Read the model definition and answer for the solid it produces. Units are mm, in the model's axes. A direction names the side the tool comes from. Give positions to 0.01 mm unless a question says otherwise; leave off trailing zeros. Order: outer loops, then holes, each group sorted by start corner. A loop starts at its lowest first (then second) coordinate and runs counter-clockwise, first axis right, second up. Notation, with made-up numbers: (86, -9.75) - (140, -9.75) arc R15 cw to (140, 18.25) - close; hole circle Ø3 at (37.25, 7.25). An arc over 180 degrees is marked (long way). Answer as CSV lines item,"result". Start each with the question number.
from build123d import *

# Parameters (mm, degrees)
EXTRUDE_1_DEPTH     = 10
CUT_EXTRUDE_1_DEPTH = 22.554195261
SKETCH_3_R          = 1.55
CUT_EXTRUDE_2_DEPTH = 10.1
CHAMFER_1_SIZE      = 2.3
SKETCH_4_W          = 6
SKETCH_4_H          = 2.8
CUT_EXTRUDE_3_DEPTH = 8.5
FILLET_1_R          = 1
CUT_EXTRUDE_4_DEPTH = 2.7
SKETCH_6_R          = 1.6
CUT_EXTRUDE_5_DEPTH = 7.3
FILLET_2_R          = 0.5


with BuildPart() as part:
    # Эскиз1 → Бобышка-Вытянуть1 (new body)
    with BuildSketch(Plane.XY):
        Polygon((7.216878365, -12.5), (14.43375673, 0), (7.216878365, 12.5), (-7.216878365, 12.5), (-14.43375673, 0), (-7.216878365, -12.5), align=None)
    extrude(amount=EXTRUDE_1_DEPTH)

    # Эскиз2 → Вырез-Вытянуть1 (cut, through all)
    with BuildSketch(Plane.XY.offset(10)):
        with BuildLine():
            Line((-2.116601049, 2.4), (2.116601049, 2.4))
            ThreePointArc((2.116601049, 2.4), (0, -3.2), (-2.116601049, 2.4))
        make_face()
    extrude(amount=-CUT_EXTRUDE_1_DEPTH, mode=Mode.SUBTRACT)

    # Эскиз3 → Вырез-Вытянуть2 (cut)
    with BuildSketch(Plane.XZ.offset(-2.4)):
        with Locations(Location((0, 5, 0), (0, 0, 270))):
            Circle(SKETCH_3_R)
    extrude(amount=-CUT_EXTRUDE_2_DEPTH, mode=Mode.SUBTRACT)

    # Фаска1
    chamfer_1_edges = [part.edges().sort_by_distance(p)[0] for p in [
        (0, 12.5, 6.55),
    ]]
    chamfer(chamfer_1_edges, length=CHAMFER_1_SIZE)

    # Эскиз4 → Вырез-Вытянуть3 (cut)
    with BuildSketch(Plane.XY.offset(10)):
        with Locations((0, 6.3)):
            Rectangle(SKETCH_4_W, SKETCH_4_H)
    extrude(amount=-CUT_EXTRUDE_3_DEPTH, mode=Mode.SUBTRACT)

    # Скругление1
    fillet_1_edges = [part.edges().sort_by_distance(p)[0] for p in [
        (10.825317547, 6.25, 10),
        (0, 12.5, 10),
        (-10.825317547, 6.25, 10),
        (-10.825317547, -6.25, 10),
        (0, -12.5, 10),
        (10.825317547, -6.25, 10),
    ]]
    fillet(fillet_1_edges, radius=FILLET_1_R)

    # Эскиз5 → Вырез-Вытянуть4 (cut)
    with BuildSketch(Plane.XY.offset(10)):
        Polygon((-11, -1.732050808), (-8, -3.464101615), (-5, -1.732050808), (-5, 1.732050808), (-8, 3.464101615), (-11, 1.732050808), align=None)
        Polygon((8, -3.464101615), (5, -1.732050808), (5, 1.732050808), (8, 3.464101615), (11, 1.732050808), (11, -1.732050808), align=None)
    extrude(amount=-CUT_EXTRUDE_4_DEPTH, mode=Mode.SUBTRACT)

    # Эскиз6 → Вырез-Вытянуть5 (cut)
    with BuildSketch(Plane.XY.offset(7.3)):
        with Locations((-8, 0)):
            Circle(SKETCH_6_R)
        with Locations((8, 0)):
            Circle(SKETCH_6_R)
    extrude(amount=-CUT_EXTRUDE_5_DEPTH, mode=Mode.SUBTRACT)

    # Скругление2
    fillet_2_edges = [part.edges().sort_by_distance(p)[0] for p in [
        (-9.6, 0, 7.3),
        (6.4, 0, 7.3),
        (3, 6.3, 10),
        (0, 7.7, 10),
        (-3, 6.3, 10),
        (0, 4.9, 10),
        (9.5, -2.598076211, 10),
        (11, 0, 10),
        (9.5, 2.598076211, 10),
        (6.5, 2.598076211, 10),
        (5, 0, 10),
        (6.5, -2.598076211, 10),
        (-11, 0, 10),
        (-9.5, -2.598076211, 10),
        (-6.5, -2.598076211, 10),
        (-5, 0, 10),
        (-6.5, 2.598076211, 10),
        (-9.5, 2.598076211, 10),
    ]]
    fillet(fillet_2_edges, radius=FILLET_2_R)


solid = part.part
(1) Straight lines are drawn through the part: line 1 (X direction, y = -0.5, z = 1); line 2 (Y direction, x = 2.75, z = 9.5); line 3 (Z direction, x = -5.75, y = 2). For each, find the intervals that lie inside material, in ascending order. Write a range as [from, to].
(2) Which of the six approach directions +Z, -Z, +X, -X, +Y, -Y give full straight-line access (tool end or side, diameter ignored) to faces 5 (the flat face through (3, 6, 6)), 6 (the flat face through (3, -2, 10))?
(3) Flat-ended cylindrical pins translate along their axes: pin 1 Ø5 at (x, z) = (0, 5) entering from +Y; pin 2 Ø5 at (y, z) = (-4, 3) entering from -X; pin 3 Ø2 at (x, y) = (-1.5, 6) entering from +Z. Find the tip coordinate at first contact, or state that the pin passes through.
(4) Determine the mould class of faces 1 (the flat face through (-10.876, -6.163, 4.437)), 2 (the cylindrical face through (0.101, -12.199, 9.715)), 3 (the cylindrical face through (10.62, -6.01, 9.71)), 4 (the flat face through (-3, 6, 6)) for opening direction X: released by +X, released by -X, zero draft, split by the parting line, or undercut.
(5) Section B-B, the plane z = 5 is taken. Write down the section's boundary in (x, y), and give its area (3 significant figures).
(6) Section A-A, the plane x = 0 is taken. Write down the section's boundary in (y, z), and give its area (3 significant figures).
(7) Section C-C, the plane y = -0.5 is taken. State how many separate pieces and enclosed holes the cut face has, and give its area (3 significant figures).
Checks:
1,line 1,"x = [-14.15, -9.52], [-6.48, -3.16], [3.16, 6.48], [9.52, 14.15]"
1,line 2,"y = [-12.37, -1.64], [1.64, 4.9], [7.7, 12.37]"
1,line 3,"z = [0, 7.3]"
2,face 5,"+Z"
2,face 6,"+Z, +X, -X, +Y, -Y"
3,pin 1,"stops at y = 11.15"
3,pin 2,"stops at x = -13.57"
3,pin 3,"stops at z = 1.5"
4,face 1,"released by -X"
4,face 2,"zero draft"
4,face 3,"released by +X"
4,face 4,"undercut"
5,outline,"(-14.43, 0) - (-7.22, -12.5) - (7.22, -12.5) - (14.43, 0) - (7.22, 12.5) - (3.85, 12.5) - (1.55, 10.2) - (1.55, 7.7) - (3, 7.7) - (3, 4.9) - (1.55, 4.9) - (1.55, 2.4) - (2.12, 2.4) arc R3.2 cw (long way) to (-2.12, 2.4) - (-1.55, 2.4) - (-1.55, 4.9) - (-3, 4.9) - (-3, 7.7) - (-1.55, 7.7) - (-1.55, 10.2) - (-3.85, 12.5) - (-7.22, 12.5) - close; hole circle Ø3.2 at (-8, 0); hole circle Ø3.2 at (8, 0)"
5,area,"451 mm²"
6,outline,"(-12.5, 0) - (-3.2, 0) - (-3.2, 10) - (-11.5, 10) arc R1 ccw to (-12.5, 9) - close; (2.4, 0) - (12.5, 0) - (12.5, 1.15) - (10.2, 3.45) - (7.7, 3.45) - (7.7, 1.5) - (4.9, 1.5) - (4.9, 3.45) - (2.4, 3.45) - close; (2.4, 6.55) - (4.9, 6.55) - (4.9, 9.5) arc R0.5 ccw to (4.4, 10) - (2.4, 10) - close; (7.7, 6.55) - (10.2, 6.55) - (12.5, 8.85) - (12.5, 9) arc R1 ccw to (11.5, 10) - (8.2, 10) arc R0.5 ccw to (7.7, 9.5) - close"
6,area,"142 mm²"
7,separate pieces,"4"
7,enclosed holes,"0"
7,area,"142 mm²"
